```python
from build123d import *

# Parameters (mm, degrees)
AUFSATZ_LINEAR_AUSTRAGEN1_DEPTH                = 43.1
SKIZZE2_R                                      = 2.55
AUFSATZ_LINEAR_AUSTRAGEN2_DEPTH                = 5
AUFSATZ_LINEAR_AUSTRAGEN2_TAPER                = 10
SCHNITT_LINEAR_AUSTRAGEN1_DEPTH                = 5.6
FASE1_SIZE                                     = 1
SCHNITT_LINEAR_AUSTRAGEN2_DEPTH                = 64.61475613
SCHNITT_LINEAR_AUSTRAGEN2_DEPTH_BACK           = 7.61475613
AUFSATZ_LINEAR_AUSTRAGEN3_DEPTH                = 30
AUFSATZ_LINEAR_AUSTRAGEN4_DEPTH                = 13
AUFSATZ_LINEAR_AUSTRAGEN5_DEPTH                = 15
AUFSATZ_LINEAR_AUSTRAGEN6_DEPTH                = 101.1
F_1_0_1_DURCHMESSER_BOHRUNG1_D                 = 1
F_1_0_1_DURCHMESSER_BOHRUNG1_DEPTH             = 25
F_1_0_1_DURCHMESSER_BOHRUNG1_TIP               = 0.30043031
F_1_0_1_DURCHMESSER_BOHRUNG2_D                 = 1
F_1_0_1_DURCHMESSER_BOHRUNG2_DEPTH             = 25
F_1_0_1_DURCHMESSER_BOHRUNG2_TIP               = 0.30043031
AUFSATZ_LINEAR_AUSTRAGEN7_DEPTH                = 5
SKIZZE48_R                                     = 28.5
SCHNITT_LINEAR_AUSTRAGEN4_DEPTH                = 6
SKIZZE49_W                                     = 58.5
SKIZZE49_H                                     = 5.6
SCHNITT_LINEAR_AUSTRAGEN8_DEPTH                = 20.5
F_6_0_6_DURCHMESSER_BOHRUNG1_D                 = 6
F_6_0_6_DURCHMESSER_BOHRUNG1_DEPTH             = 5
AUFSATZ_LINEAR_AUSTRAGEN8_DEPTH                = 5.864512
AUFSATZ_LINEAR_AUSTRAGEN9_DEPTH                = 5.865
SCHNITT_LINEAR_AUSTRAGEN11_DEPTH               = 22
F_4_0_4_DURCHMESSER_BOHRUNG2_D                 = 4
F_4_0_4_DURCHMESSER_BOHRUNG2_DEPTH             = 6
STIRNSENKUNG_F_R_M5_ZYLINDERSCHRAUBE_3_A_COUNT = 2
STIRNSENKUNG_F_R_M5_ZYLINDERSCHRAUBE_3_A_PITCH = 64.5


with BuildPart() as part:
    # Skizze1 → Aufsatz-Linear austragen1 (new body)
    with BuildSketch(Plane.XY):
        with BuildLine():
            Line((27.11475613, -10), (35.11475613, -10))
            Line((35.11475613, -10), (35.11475613, -35))
            Line((35.11475613, -35), (-35.11475613, -35))
            Line((-35.11475613, -35), (-35.11475613, -10))
            Line((-35.11475613, -10), (-27.11475613, -10))
            ThreePointArc((-27.11475613, -10), (0, -28.9), (27.11475613, -10))
        make_face()
    extrude(amount=AUFSATZ_LINEAR_AUSTRAGEN1_DEPTH)

    # Skizze2 → Aufsatz-Linear austragen2 (add)
    with BuildSketch(Plane(origin=(0, 0, 0), x_dir=(-1, 0, 0), z_dir=(0, 0, -1))):
        with Locations((-23.5, -23.663738082)):
            Circle(SKIZZE2_R)
        with Locations((23.5, -23.663738082)):
            Circle(SKIZZE2_R)
    extrude(amount=AUFSATZ_LINEAR_AUSTRAGEN2_DEPTH, taper=AUFSATZ_LINEAR_AUSTRAGEN2_TAPER)

    # Skizze3 → Schnitt-Linear austragen1 (cut)
    with BuildSketch(Plane.XY.offset(43.1)):
        with BuildLine():
            Line((28.5, -23.663738082), (28.5, -7.705302488))
            Line((28.5, -7.705302488), (-28.5, -7.705302488))
            Line((-28.5, -7.705302488), (-28.5, -23.663738082))
            ThreePointArc((-28.5, -23.663738082), (-23.5, -28.663738082), (-18.5, -23.663738082))
            Line((-18.5, -23.663738082), (-18.5, -22.202702538))
            Line((-18.5, -22.202702538), (18.5, -22.202702538))
            Line((18.5, -22.202702538), (18.5, -23.663738082))
            ThreePointArc((18.5, -23.663738082), (23.5, -28.663738082), (28.5, -23.663738082))
        make_face()
    extrude(amount=-SCHNITT_LINEAR_AUSTRAGEN1_DEPTH, mode=Mode.SUBTRACT)

    # Fase1
    fase1_edges = [part.edges().sort_by_distance(p)[0] for p in [
        (27.807378065, -10, 37.5),
        (-27.807378065, -10, 37.5),
    ]]
    chamfer(fase1_edges, length=FASE1_SIZE)

    # Skizze4 → Schnitt-Linear austragen2 (cut, two sides)
    with BuildSketch(Plane(origin=(-28.5, 0, 0), x_dir=(0, 0, -1), z_dir=(1, 0, 0))) as schnitt_linear_austragen2_sk:
        Polygon((-36.5, -10), (-37.5, -11), (-37.5, -23.663738082), (-43.1, -23.663738082), (-43.1, -10), align=None)
    extrude(amount=SCHNITT_LINEAR_AUSTRAGEN2_DEPTH, mode=Mode.SUBTRACT)
    extrude(schnitt_linear_austragen2_sk.sketch, amount=-SCHNITT_LINEAR_AUSTRAGEN2_DEPTH_BACK, mode=Mode.SUBTRACT)

    # Skizze5 → Aufsatz-Linear austragen3 (add)
    with BuildSketch(Plane.XY.offset(43.1)):
        Polygon((-35.11475613, -35), (-35.11475613, -23.663738082), (-31.11475613, -23.663738082), (-31.11475613, -31), (31.11475613, -31), (31.11475613, -23.663738082), (35.11475613, -23.663738082), (35.11475613, -35), align=None)
    extrude(amount=AUFSATZ_LINEAR_AUSTRAGEN3_DEPTH)

    # Skizze6 → Aufsatz-Linear austragen4 (add)
    with BuildSketch(Plane.XY.offset(73.1)):
        with BuildLine():
            Line((35.11475613, -35), (-35.11475613, -35))
            Line((-35.11475613, -35), (-35.11475613, -20))
            Line((-35.11475613, -20), (-20.303940504, -20))
            ThreePointArc((-20.303940504, -20), (0, -28.5), (20.303940504, -20))
            Line((20.303940504, -20), (35.11475613, -20))
            Line((35.11475613, -20), (35.11475613, -35))
        make_face()
    extrude(amount=AUFSATZ_LINEAR_AUSTRAGEN4_DEPTH)

    # Skizze7 → Aufsatz-Linear austragen5 (add)
    with BuildSketch(Plane.XY.offset(86.1)):
        with BuildLine():
            Line((35.11475613, -35), (-35.11475613, -35))
            Line((-35.11475613, -35), (-35.11475613, -20))
            Line((-35.11475613, -20), (-20.444070045, -20))
            ThreePointArc((-20.444070045, -20), (0, -28.6), (20.444070045, -20))
            Line((20.444070045, -20), (35.11475613, -20))
            Line((35.11475613, -20), (35.11475613, -35))
        make_face()
    extrude(amount=AUFSATZ_LINEAR_AUSTRAGEN5_DEPTH)

    # Skizze24 → Aufsatz-Linear austragen6 (add)
    with BuildSketch(Plane(origin=(0, 0, 0), x_dir=(-1, 0, 0), z_dir=(0, 0, -1))):
        Polygon((-8.62, -41), (-14.62, -35), (21.38, -35), (15.38, -41), align=None)
    extrude(amount=-AUFSATZ_LINEAR_AUSTRAGEN6_DEPTH)

    # Ø1.0 (1) Durchmesser Bohrung1
    with Locations(Plane(origin=(0, -41, 0), x_dir=(-1, 0, 0), z_dir=(0, -1, 0))):
        with Locations((3.38, -25)):
            Hole(F_1_0_1_DURCHMESSER_BOHRUNG1_D / 2, depth=F_1_0_1_DURCHMESSER_BOHRUNG1_DEPTH)
            with Locations((0, 0, -(F_1_0_1_DURCHMESSER_BOHRUNG1_DEPTH + F_1_0_1_DURCHMESSER_BOHRUNG1_TIP / 2))):  # 118° drill point
                Cone(0, F_1_0_1_DURCHMESSER_BOHRUNG1_D / 2, F_1_0_1_DURCHMESSER_BOHRUNG1_TIP, mode=Mode.SUBTRACT)

    # Skizze32 → Stirnsenkung f_r M5 Zylinderschraube mit (revolve, cut)
    with BuildSketch(Plane(origin=(-3.38, -28.9, 25), x_dir=(0, 0, -1), z_dir=(1, 0, 0))):
        Polygon((0, 0), (0, 26.652366702), (2.75, 25), (2.75, 7), (5.4, 7), (5.4, 0), align=None)
    revolve(axis=Axis((-3.38, -35.25, 25), (0, 1, 0)), mode=Mode.SUBTRACT)

    # Ø1.0 (1) Durchmesser Bohrung2
    with Locations(Plane(origin=(0, -41, 0), x_dir=(-1, 0, 0), z_dir=(0, -1, 0))):
        with Locations((3.38, -90)):
            Hole(F_1_0_1_DURCHMESSER_BOHRUNG2_D / 2, depth=F_1_0_1_DURCHMESSER_BOHRUNG2_DEPTH)
            with Locations((0, 0, -(F_1_0_1_DURCHMESSER_BOHRUNG2_DEPTH + F_1_0_1_DURCHMESSER_BOHRUNG2_TIP / 2))):  # 118° drill point
                Cone(0, F_1_0_1_DURCHMESSER_BOHRUNG2_D / 2, F_1_0_1_DURCHMESSER_BOHRUNG2_TIP, mode=Mode.SUBTRACT)

    # Skizze41 → Stirnsenkung f_r M5 Zylinderschraube 2 (revolve, cut)
    with BuildSketch(Plane(origin=(-3.38, -28.6, 90), x_dir=(0, 0, -1), z_dir=(1, 0, 0))):
        Polygon((0, 0), (0, 26.652366702), (2.75, 25), (2.75, 7), (5.4, 7), (5.4, 0), align=None)
    revolve(axis=Axis((-3.38, -34.95, 90), (0, 1, 0)), mode=Mode.SUBTRACT)

    # Skizze45 → Aufsatz-Linear austragen7 (add)
    with BuildSketch(Plane(origin=(0, 0, 0), x_dir=(-1, 0, 0), z_dir=(0, 0, -1))):
        Polygon((-35.11475613, -35), (-14.62, -35), (-8.62, -41), (15.38, -41), (21.38, -35), (35.11475613, -35), (35.11475613, 35.295549341), (-35.11475613, 35.295549341), align=None)
    extrude(amount=AUFSATZ_LINEAR_AUSTRAGEN7_DEPTH)

    # Skizze48 → Schnitt-Linear austragen4 (cut, through all)
    with BuildSketch(Plane.XY):
        Circle(SKIZZE48_R)
    extrude(amount=-SCHNITT_LINEAR_AUSTRAGEN4_DEPTH, mode=Mode.SUBTRACT)

    # Skizze49 → Schnitt-Linear austragen8 (cut)
    with BuildSketch(Plane(origin=(0, -10, 0), x_dir=(1, 0, 0), z_dir=(0, 1, 0))):
        with Locations((-0.00024387, -2.8)):
            Rectangle(SKIZZE49_W, SKIZZE49_H)
    extrude(amount=-SCHNITT_LINEAR_AUSTRAGEN8_DEPTH, mode=Mode.SUBTRACT)

    # Ø6.0 (6) Durchmesser Bohrung1
    with Locations(Plane(origin=(0, 0, -5), x_dir=(-1, 0, 0), z_dir=(0, 0, -1))):
        with Locations((-23.752539123, 23.39599293), (23.752539123, 23.39599293), (23.752539123, -23.39599293), (-23.752539123, -23.39599293)):
            Hole(F_6_0_6_DURCHMESSER_BOHRUNG1_D / 2, depth=F_6_0_6_DURCHMESSER_BOHRUNG1_DEPTH)

    # Skizze54 → Aufsatz-Linear austragen8 (add)
    with BuildSketch(Plane.ZY.offset(35.11475613)):
        Polygon((0, 35.295549341), (36.5, -10), (0, -10), align=None)
    extrude(amount=-AUFSATZ_LINEAR_AUSTRAGEN8_DEPTH)

    # Skizze55 → Aufsatz-Linear austragen9 (add)
    with BuildSketch(Plane(origin=(35.11475613, 0, 0), x_dir=(0, 0, -1), z_dir=(1, 0, 0))):
        Polygon((0, 35.295549341), (0, -10), (-36.5, -10), align=None)
    extrude(amount=-AUFSATZ_LINEAR_AUSTRAGEN9_DEPTH)

    # Skizze62 → Schnitt-Linear austragen11 (cut)
    with BuildSketch(Plane.XY.offset(101.1)):
        Polygon((-35.11475613, -20), (-27.779413088, -20), (-21.38, -35), (-35.11475613, -35), align=None)
        Polygon((35.11475613, -20), (27.779413088, -20), (14.62, -35), (35.11475613, -35), align=None)
    extrude(amount=-SCHNITT_LINEAR_AUSTRAGEN11_DEPTH, mode=Mode.SUBTRACT)

    # Ø4.0 (4) Durchmesser Bohrung2
    with Locations(Plane.XY.offset(79.1)):
        with Locations((-30, -25), (30, -25)):
            Hole(F_4_0_4_DURCHMESSER_BOHRUNG2_D / 2, depth=F_4_0_4_DURCHMESSER_BOHRUNG2_DEPTH)

    # Skizze68 → Stirnsenkung f_r M5 Zylinderschraube 3 (revolve, cut)
    with BuildSketch(Plane(origin=(-3.38, -28.6, 25), x_dir=(0, 0, 1), z_dir=(1, 0, 0))):
        Polygon((0, 0), (0, 26.59228064), (2.65, 25), (2.65, 6), (5.4, 6), (5.4, 0), align=None)
    stirnsenkung_f_r_m5_zylinderschraube_3 = revolve(axis=Axis((-3.38, -22.25, 25), (0, -1, 0)), mode=Mode.SUBTRACT)

    # Stirnsenkung f_r M5 Zylinderschraube 3 a: Stirnsenkung f_r M5 Zylinderschraube 3 ×2
    with Locations(*[(0, 0, i * STIRNSENKUNG_F_R_M5_ZYLINDERSCHRAUBE_3_A_PITCH) for i in range(1, STIRNSENKUNG_F_R_M5_ZYLINDERSCHRAUBE_3_A_COUNT)]):
        add(stirnsenkung_f_r_m5_zylinderschraube_3, mode=Mode.SUBTRACT)


solid = part.part
```
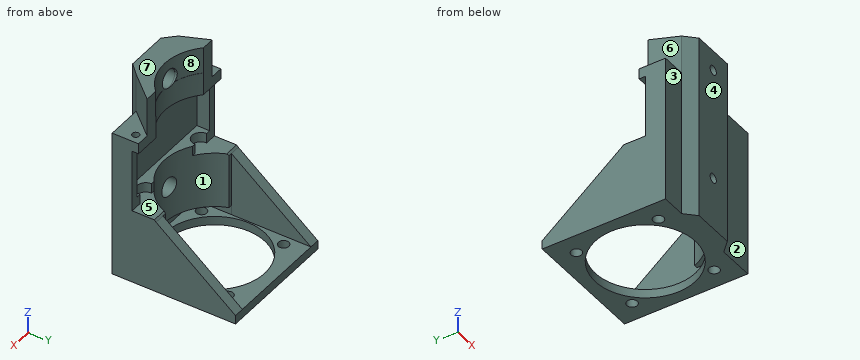
For this review, take the finished solid that the model builds, in its own axes (mm). Face numbers are marked on the shaded views. A direction names the side the tool comes from. Coordinates: 2 decimals unless noted, no trailing zeros. Order: outer loops, then holes, each group sorted by start corner. A loop starts at its lowest first (then second) coordinate and runs counter-clockwise, first axis right, second up. Notation, with made-up numbers: (54.5, 87) -> (60.5, 87) arc R10 ccw to (60.5, 95) -> close; hole circle Ø3 at (-36.75, 42). An arc over 180 degrees is marked (long way). Use CSV: the item, a comma, the result in double quotes. Start each with the question number.
Item 1: Insertion check: pin 1 (2 mm diameter, centred on x = 17.5, z = 40.5, fed in from +Y); pin 2 (12 mm diameter, centred on x = -31, z = 86.5, fed in from +Y); pin 3 (8 mm diameter, centred on x = -14, z = 21, fed in from +Y). Each pin has a flat end and moves straight along its axis. Give the tip position at first contact, or say it passes through.
Item 2: We need section D-D, the plane y = -17.5. Give the boundary of the cut face in (x, z), then the cut area to 3 significant figures.
Item 3: Wall thickness on probe 1 along Z at (x, y) = (-3.38, -38.75); probe 2 along Y at (x, z) = (30, 77.05); probe 3 along X at (y, z) = (14.5, 7.5): over which ranges is each line inside the solid? List them lowest first.
Item 4: We need section A-A, the plane y = 18.5. Give the boundary of the cut face in (x, z), then the cut area to 3 significant figures.
Item 5: We need section B-B, the plane z = 46. Give the boundary of the cut face in (x, y).
Item 6: We need section C-C, the plane x = 23.5. Give the boundary of the cut face in (y, z), then the cut area to 3 significant figures.
Item 7: Draft analysis for pull direction X (two halves, no side actions). For the marked faces 5, 6, 7 and 8, state which applies: pulls with the +X half, pulls with the -X half, needs draft (parallel to the pull), parting line crosses it, or undercut.
Item 8: For the marked faces 1, 2, 3 and 4, list the 3-axis set-ups (+Z, -Z, +X, -X, +Y, -Y) from which the entire face can be reached by the end or side of a thin tool; tool diameter is ignored.
Derived:
1,pin 1,"stops at y = -23.66"
1,pin 2,"stops at y = -20"
1,pin 3,"stops at y = -22.61"
2,outline,"(-35.11, -5) -> (-22.49, -5) -> (-22.49, 0) -> (-29.25, 0) -> (-29.25, 5.6) -> (-23, 5.6) -> (-23, 37.5) -> (-35.11, 37.5) -> close; (22.49, -5) -> (35.11, -5) -> (35.11, 37.5) -> (23, 37.5) -> (23, 5.6) -> (29.25, 5.6) -> (29.25, 0) -> (22.49, 0) -> close"
2,area,"965 mm^2"
3,probe 1,"z = -5 to 22.35, 27.65 to 86.85, 92.15 to 101.1"
3,probe 2,"y = -35 to -27, -23 to -20"
3,probe 3,"x = -35.11 to -29.25, 29.25 to 35.11"
4,outline,"(-35.11, -5) -> (-21.68, -5) -> (-21.68, 0) -> (-29.25, 0) -> (-29.25, 13.53) -> (-35.11, 13.53) -> close; (21.68, -5) -> (35.11, -5) -> (35.11, 13.53) -> (29.25, 13.53) -> (29.25, 0) -> (21.68, 0) -> close"
4,area,"293 mm^2"
5,outline,"(-35.11, -35) -> (-21.38, -35) -> (-15.38, -41) -> (8.62, -41) -> (14.62, -35) -> (35.11, -35) -> (35.11, -23.66) -> (31.11, -23.66) -> (31.11, -31) -> (-31.11, -31) -> (-31.11, -23.66) -> (-35.11, -23.66) -> close"
6,outline,"(-35, -5) -> (-26.39, -5) -> (-26.39, 0) -> (-30.5, 0) -> (-30.5, 5.6) -> (-16.82, 5.6) -> (-16.82, 37.5) -> (-28.66, 37.5) -> (-28.66, 43.1) -> (-31, 43.1) -> (-31, 73.1) -> (-20, 73.1) -> (-20, 101.1) -> (-24.88, 101.1) -> (-24.88, 79.1) -> (-35, 79.1) -> close; (-20.41, -5) -> (-16.12, -5) -> (-16.12, 0) -> (-20.41, 0) -> close; (16.12, -5) -> (20.41, -5) -> (20.41, 0) -> (16.12, 0) -> close; (26.39, -5) -> (35.3, -5) -> (35.3, 0) -> (26.39, 0) -> close"
6,area,"1,090 mm^2"
7,face 5,"undercut"
7,face 6,"pulls with the -X half"
7,face 7,"needs draft"
7,face 8,"undercut"
8,face 1,"+Y"
8,face 2,"+Z, -Z, +X, -Y"
8,face 3,"+Z, -Z, -X, -Y"
8,face 4,"+Z, -Z, +X, -X, -Y"
